Check sheet for the modelled part. Datum: model origin and axes. Units: mm. Face numbers are marked on the shaded views. A direction names the side the tool comes from. Give positions to 0.01 mm unless a question says otherwise; leave off trailing zeros. Write each loop counter-clockwise with the first axis right and the second up, starting at its lowest first coordinate (ties: lowest second). Pieces come first, ordered by that corner, then holes. Notation, with made-up numbers: M 81.5,-15 L 91.5,-15 A20 cw 91.5,0 Z; hole C 63,61 d11. An arc over 180 degrees is marked long. Write each question's results on one line, items separated by ' | '. Start each with the question number.
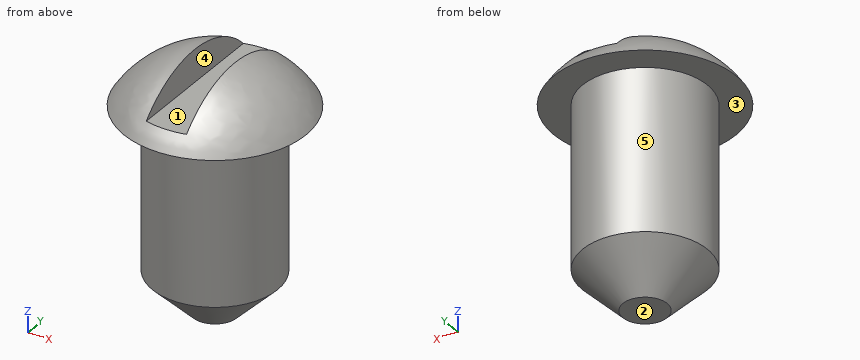
from build123d import *

# Parameters (mm, degrees)
F3_W     = 2.54
F3_H     = 10.16
F4_DEPTH = 25.4
F5_SIZE  = 2.54


with BuildPart() as f1:
    # F0 (on Front) → F1 (revolve)
    with BuildSketch(Plane.XZ):
        with BuildLine():
            Line((0, 9.113751), (0, 0))
            Line((0, 0), (3.932627, 0))
            Line((3.932627, 0), (3.932627, 12.7))
            Line((3.932627, 12.7), (5.73178, 12.7))
            ThreePointArc((5.73178, 12.7), (3.276199, 15.028225), (0, 15.875))
            Line((0, 15.875), (0, 9.113751))
        make_face()
    revolve(axis=Axis((0, 0, -3.129652), (0, 0, -1)))

    # F3 (on offset) → F4 (cut)
    with BuildSketch(Plane.XY.offset(13.716)):
        Rectangle(F3_W, F3_H)
    extrude(amount=F4_DEPTH, mode=Mode.SUBTRACT)

    # F5
    f5_edges = [f1.edges().sort_by_distance(p)[0] for p in [
        (-3.932627, 0, 0),
    ]]
    chamfer(f5_edges, length=F5_SIZE)


solid = f1.part
Q1. Scan lines: L1, parallel to Z at x = 0.5, y = 0.5; L2, parallel to X at y = 0, z = 9; L3, parallel to Y at x = 0.5, z = 9.75. Record each from-to range of solid material in increasing order.
Q2. Depth check by flat-ended pin: pin 1 Ø1.6 at (y, z) = (0, 15) entering from -X; pin 2 Ø6 at (y, z) = (-3.5, 11) entering from -X; pin 3 Ø2 at (x, y) = (-3, -1.5) entering from -Z. Enter the tip coordinate at first touch or a pass-through.
Q3. Section check A-A on z = 9.25. Record the boundary of the cut face in (x, y).
Q4. Tool access check on the marked faces 1 and 2. Record the directions out of +Z, -Z, +X, -X, +Y, -Y that give a thin tool (end or side, any length) a straight path to the whole face; none if there is none.
Q5. Release check for a two-part mould opening along X. For the marked faces 3, 4 and 5 record: pulls with the +X half, pulls with the -X half, needs draft (parallel to the pull), parting line crosses it, or undercut.
Check result:
1) L1: 0 to 13.72 | L2: -3.93 to 3.93 | L3: -3.9 to 3.9
2) pin 1: x = -4.45 | pin 2: x = -5.64 | pin 3: z = 0.96
3) outline: C 0,0 d7.87
4) face 1: +Z, +Y, -Y | face 2: -Z, +X, -X, +Y, -Y
5) face 3: needs draft | face 4: undercut | face 5: parting line crosses it
